Design review of the part built by this model. Coordinates are the model's own, in mm. Face numbers are marked on the shaded views. Coordinates: 2 decimals unless noted, no trailing zeros. Order: outer loops, then holes, each group sorted by start corner. A loop starts at its lowest first (then second) coordinate and runs counter-clockwise, first axis right, second up. Notation, with made-up numbers: (83.25, 21) - (139.25, 21) arc R22 ccw to (139.25, 48) - close; hole circle Ø1 at (16.5, 63). An arc over 180 degrees is marked (long way). Write each question's results on one line, items separated by ' | '. Start each with the question number.
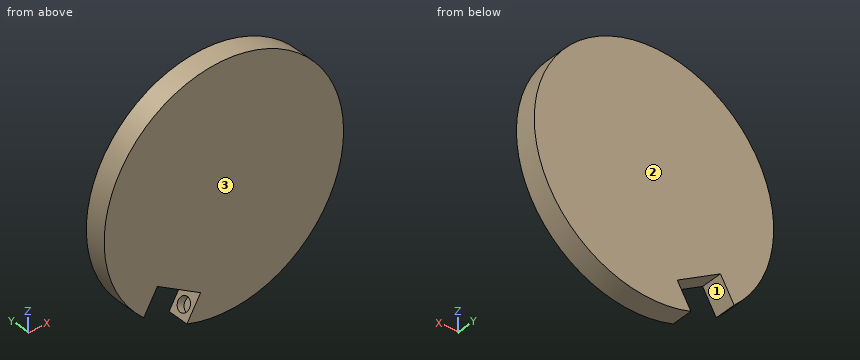
```python
from build123d import *

# Parameters (mm, degrees)
BOSS_EXTRUDE1_DEPTH      = 13.9999974
BOSS_EXTRUDE1_DEPTH_BACK = 13.9999974
SKETCH4_R                = 152.4
CUT_EXTRUDE2_DEPTH       = 218.337340806
CUT_EXTRUDE2_DEPTH_BACK  = 218.337340806
SKETCH9_R                = 8.89
CUT_EXTRUDE4_DEPTH       = 41.91


with BuildPart() as part:
    # Sketch4 → Boss-Extrude1 (new, two sides: drawn at the far end of the back side and taken through both)
    with BuildSketch(Plane(origin=(0, 0, 0), x_dir=(1, 0, 0), z_dir=(0, 1, 0)).offset(-BOSS_EXTRUDE1_DEPTH_BACK)):
        with Locations(Location((0, 0, 0), (0, 0, 270))):
            Circle(SKETCH4_R)
    extrude(amount=BOSS_EXTRUDE1_DEPTH + BOSS_EXTRUDE1_DEPTH_BACK)

    # Sketch7 → Cut-Extrude2 (cut, two sides: drawn at the far end of the back side and taken through both)
    with BuildSketch(Plane(origin=(0, 13.9999974, 0), x_dir=(1, 0, 0), z_dir=(0, 1, 0)).offset(-CUT_EXTRUDE2_DEPTH_BACK)):
        Polygon((-48.70369343, 147.857271537), (-103.69630657, 116.107271537), (-84.64630657, 83.111703653), (-29.65369343, 114.861703653), align=None)
    extrude(amount=CUT_EXTRUDE2_DEPTH + CUT_EXTRUDE2_DEPTH_BACK, mode=Mode.SUBTRACT)

    # Sketch9 → Cut-Extrude4 (cut)
    with BuildSketch(Plane(origin=(0, 0, 0), x_dir=(-0.500000000000002, 0, -0.8660254037844375), z_dir=(0.8660254037844375, 0, -0.500000000000002))):
        with Locations((134.218010674, 0)):
            Circle(SKETCH9_R)
    extrude(amount=CUT_EXTRUDE4_DEPTH, mode=Mode.SUBTRACT)


solid = part.part
```
(1) Take a section at D-D (z = -27.5). State the section outline as (x, y) points, plus the area to 3 significant figures.
(2) Clearance check with flat-ended pins moving along their axes: pin 1 (1.5 mm diameter, centred on y = -0.5, z = -121, fed in from -X); pin 2 (6 mm diameter, centred on y = 10, z = 113, fed in from -X); pin 3 (3 mm diameter, centred on x = 84.5, y = -6, fed in from -Z). State where each tip first meets the part, or that it passes through.
(3) Take a section at B-B (y = -4.5). State the section outline as (x, z) points, plus the area to 3 significant figures.
(4) Take a section at C-C (x = 129). State the section outline as (y, z) points.
(5) To check wall thickness, follow line 1 along X through (y, z) = (-4, -100.5); line 2 along X through (y, z) = (9.5, -105); line 3 along Z through (x, y) = (1, 11). State the ranges of each line that lie inside material, in increasing order. Write a range as [from, to].
(6) Mouldability with a two-part tool opening along Y and no side actions: class the marked faces 1, 2 and 3 as +Y half, -Y half, draft (parallel to the pull), parting line (faces both ways), or undercut.
(7) Take a section at A-A (z = -102). State the section outline as (x, y) points, plus the area to 3 significant figures.
Worked out:
1) outline: (-149.9, -14) - (149.9, -14) - (149.9, 14) - (-149.9, 14) - close | area: 8,390 mm^2
2) pin 1: x = -33.63 | pin 2: x = -105.48 | pin 3: z = -127.82
3) outline: (-102.02, -113.21) - (-84.65, -83.11) - (-29.65, -114.86) - (-35.78, -125.47) - (-26.98, -130.55) - (-34.65, -143.83) - (-43.45, -138.75) - (-47.03, -144.96) arc R152.4 ccw (long way) to start | area: 70,500 mm^2
4) outline: (-14, -81.15) - (14, -81.15) - (14, 81.15) - (-14, 81.15) - close
5) line 1: [-114.57, -94.69], [-54.53, 114.57] | line 2: [-110.46, -97.28], [-46.73, 110.46] | line 3: [-152.4, 152.4]
6) face 1: draft | face 2: +Y half | face 3: -Y half
7) outline: (-113.23, -14) - (-95.55, -14) - (-95.55, 14) - (-113.23, 14) - close; (-51.93, -14) - (113.23, -14) - (113.23, 14) - (-51.93, 14) - close | area: 5,120 mm^2
